Build history of the part. All positions in model axes, mm. Face numbers are marked on the shaded views. A direction names the side the tool comes from. Round coordinates to 2 decimals unless told otherwise and drop trailing zeros. Loops run counter-clockwise (first coordinate to the right, second up) from the corner with the lowest first, then second, coordinate; pieces in that order, holes last. Notation, with made-up numbers: (11, 55.25) - (27, 55.25) arc R20 cw to (27, 92.25) - close; hole circle Ø8 at (-0.75, 17). An arc over 180 degrees is marked (long way). Put each result on its own line as item: value. Start each with the question number.
from build123d import *

# Parameters (mm, degrees)
SKETCH_1_R               = 5.1
SKETCH_1_R_2             = 2.6
EXTRUDE_1_DEPTH          = 15
CUT_EXTRUDE_1_DEPTH      = 17.643917808
CUT_EXTRUDE_1_DEPTH_BACK = 17.643917808
SKETCH_2_R               = 1.35
CUT_EXTRUDE_2_DEPTH      = 17.643917959
CUT_EXTRUDE_2_DEPTH_BACK = 17.643917959
SKETCH_3_R               = 1.35
SKETCH_4_R               = 12.5
SKETCH_4_R_2             = 1.65
EXTRUDE_2_DEPTH          = 3


with BuildPart() as part:
    # 草图1 → 凸台-拉伸1 (new body)
    with BuildSketch(Plane.XY):
        Circle(SKETCH_1_R)
        Circle(SKETCH_1_R_2, mode=Mode.SUBTRACT)
    extrude(amount=EXTRUDE_1_DEPTH)

    # 草图2 → 切除-拉伸1 (cut, two sides: drawn at the far end of the back side and taken through both)
    with BuildSketch(Plane(origin=(0, 0, 0), x_dir=(1, 0, 0), z_dir=(0, 1, 0)).offset(-CUT_EXTRUDE_1_DEPTH_BACK)):
        with Locations(Location((0, -5, 0), (0, 0, 90))):
            Circle(SKETCH_2_R)
    extrude(amount=CUT_EXTRUDE_1_DEPTH + CUT_EXTRUDE_1_DEPTH_BACK, mode=Mode.SUBTRACT)

    # 草图3 → 切除-拉伸2 (cut, two sides: drawn at the far end of the back side and taken through both)
    with BuildSketch(Plane(origin=(0, 0, 0), x_dir=(0, 0, -1), z_dir=(1, 0, 0)).offset(-CUT_EXTRUDE_2_DEPTH_BACK)):
        with Locations((-5, 0)):
            Circle(SKETCH_3_R)
    extrude(amount=CUT_EXTRUDE_2_DEPTH + CUT_EXTRUDE_2_DEPTH_BACK, mode=Mode.SUBTRACT)

    # 草图4 → 凸台-拉伸2 (add)
    with BuildSketch(Plane.XY):
        Circle(SKETCH_4_R)
        with Locations((0, -10)):
            Circle(SKETCH_4_R_2, mode=Mode.SUBTRACT)
        with Locations((-10, 0)):
            Circle(SKETCH_4_R_2, mode=Mode.SUBTRACT)
        with Locations((0, 10)):
            Circle(SKETCH_4_R_2, mode=Mode.SUBTRACT)
        with Locations((10, 0)):
            Circle(SKETCH_4_R_2, mode=Mode.SUBTRACT)
    extrude(amount=-EXTRUDE_2_DEPTH)


solid = part.part
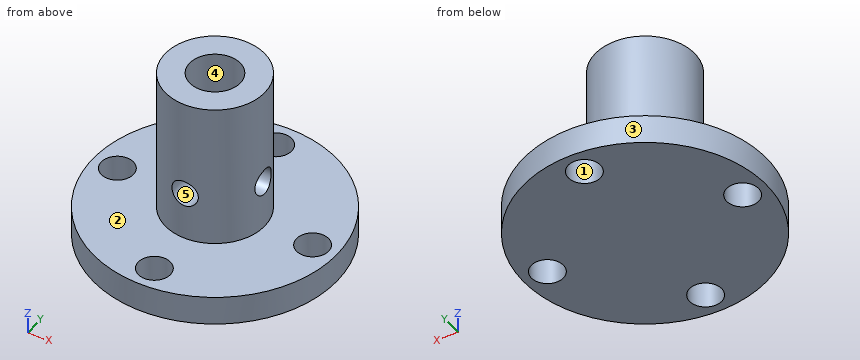
Item 1: Slice it at A-A (y = -10). Give the cut face in (x, z), plus the area to 3 significant figures.
Item 2: Slice it at D-D (x = 0). Give the cut face in (y, z), plus the area to 3 significant figures.
Item 3: Two-plate mould, pull along X, no slides. Class the marked faces 1, 2 and 3: pulls with the +X half, pulls with the -X half, needs draft (parallel to the pull), parting line crosses it, or undercut.
Item 4: Drill centre lines: probe 1 along Y at (x, z) = (0, -1.7); probe 2 along Z at (x, y) = (3.3, 0); probe 3 along Y at (x, z) = (0, 8.25). Where is each one in solid material? Low to high. Write a range as [from, to].
Item 5: Slice it at C-C (z = 6). Give the cut face in (x, y).
Item 6: Drop flat-ended pins along their axis: pin 1 Ø10 at (y, z) = (-8.5, 0) entering from -X; pin 2 Ø2 at (x, z) = (-1, 2.5) entering from +Y; pin 3 Ø2 at (x, y) = (-10, 0) entering from -Z; pin 4 Ø3 at (y, z) = (0, 5) entering from +X. Give the stop position or say it passes through.
Item 7: Which spindle directions (+Z, -Z, +X, -X, +Y, -Y) get a long thin tool onto all of the face, cutting with end or side? Do the marked faces 4 and 5. Say none if no direction does.
Computed values:
1. outline: (-7.5, -3) - (-1.65, -3) - (-1.65, 0) - (-7.5, 0) - close; (1.65, -3) - (7.5, -3) - (7.5, 0) - (1.65, 0) - close
1. area: 35.1 mm^2
2. outline: (-12.5, -3) - (-11.65, -3) - (-11.65, 0) - (-12.5, 0) - close; (-8.35, -3) - (8.35, -3) - (8.35, 0) - (5.1, 0) - (5.1, 3.65) - (2.6, 3.65) - (2.6, 0) - (-2.6, 0) - (-2.6, 3.65) - (-5.1, 3.65) - (-5.1, 0) - (-8.35, 0) - close; (-5.1, 6.35) - (-2.6, 6.35) - (-2.6, 15) - (-5.1, 15) - close; (2.6, 6.35) - (5.1, 6.35) - (5.1, 15) - (2.6, 15) - close; (11.65, -3) - (12.5, -3) - (12.5, 0) - (11.65, 0) - close
2. area: 117 mm^2
3. face 1: undercut
3. face 2: needs draft
3. face 3: parting line crosses it
4. probe 1: y = [-12.5, -11.65], [-8.35, 8.35], [11.65, 12.5]
4. probe 2: z = [-3, 3.65], [6.35, 15]
4. probe 3: y = [-5.1, -2.6], [2.6, 5.1]
5. outline: (-5.02, -0.91) arc R5.1 ccw to (-0.91, -5.02) - (-0.91, -2.44) arc R2.6 cw to (-2.44, -0.91) - close; (-5.02, 0.91) - (-2.44, 0.91) arc R2.6 cw to (-0.91, 2.44) - (-0.91, 5.02) arc R5.1 ccw to start; (0.91, -5.02) arc R5.1 ccw to (5.02, -0.91) - (2.44, -0.91) arc R2.6 cw to (0.91, -2.44) - close; (0.91, 2.44) arc R2.6 cw to (2.44, 0.91) - (5.02, 0.91) arc R5.1 ccw to (0.91, 5.02) - close
6. pin 1: stops at x = -12
6. pin 2: stops at y = 5.1
6. pin 3: passes through
6. pin 4: stops at x = 5.1
7. face 4: +Z
7. face 5: +Y, -Y
